Geometry: see drawing. Coordinates: mm, zero at the bounding-box minimum. A direction names the side the tool comes from. Coordinates: 2 decimals unless noted, no trailing zeros. Loops run counter-clockwise (first coordinate to the right, second up) from the corner with the lowest first, then second, coordinate; pieces in that order, holes last. Notation, with made-up numbers: (-26.75, 14.5) -> (-9.75, 14.5) arc R16 ccw to (-9.75, 31.5) -> close; hole circle Ø10 at (-6, 38). An arc over 180 degrees is marked (long way). Answer as a JSON object with one key per item and string values.
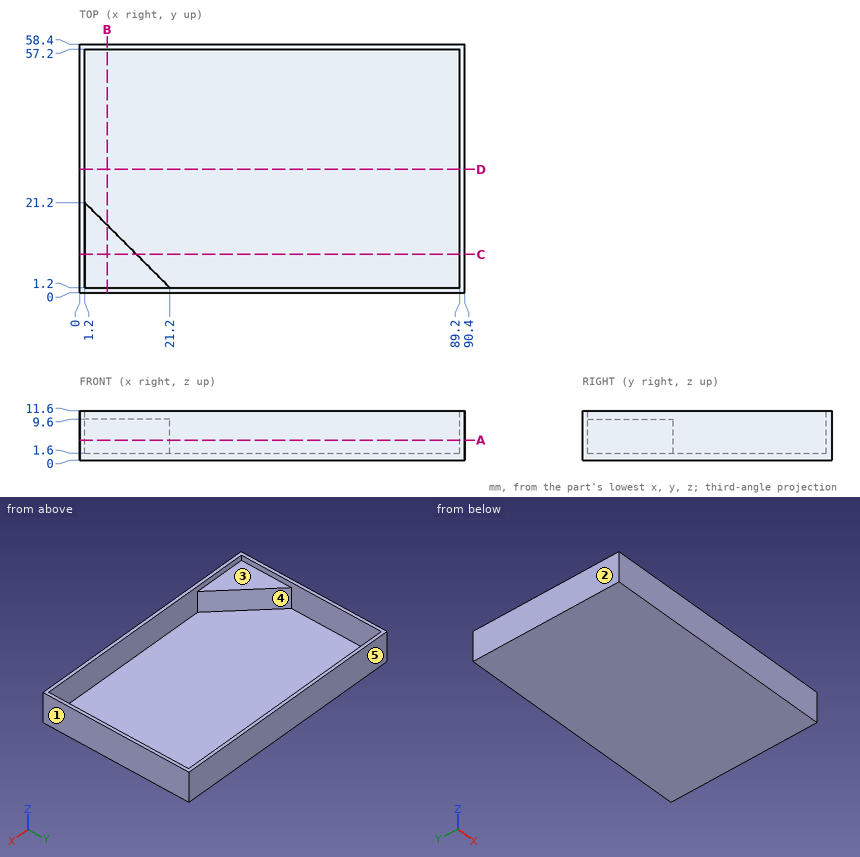
1. Mould query, pull axis X, two halves, no side actions, for the marked faces 1, 2 and 3. Classes: pulls with the +X half, pulls with the -X half, needs draft (parallel to the pull), parting line crosses it, or undercut.
Reply:
{"face 1": "pulls with the +X half", "face 2": "pulls with the -X half", "face 3": "undercut"}
2. Pin query (flat end, axial travel): P1, Ø3, axis at y = 47, z = 4, coming from the -X side; P2, Ø8, axis at x = 43, y = 11, coming from the +Z side; P3, Ø6, axis at x = 8, y = 9, coming from the +Z side. Return the tip coordinate at first contact, or that it passes through.
Reply:
{"P1": "stops at x = 0", "P2": "stops at z = 1.6", "P3": "stops at z = 9.6"}
3. Access query for the marked faces 4 and 5. Directions: +Z, -Z, +X, -X, +Y, -Y. A direction counts if a zero-diameter tool reaches every point of the face in a straight line with its end or side. Return the directions, or none.
Reply:
{"face 4": "+Z", "face 5": "+Z, -Z, +X, -X, +Y"}
4. Line query: line 1 along Y through (x, z) = (43, 9); line 2 along X through (y, z) = (36.5, 5.75); line 3 along Z through (x, y) = (61.5, 39). Output: solid intervals per line, ascending.
Reply:
{"line 1": "y = 0 to 1.2, 57.2 to 58.4", "line 2": "x = 0 to 1.2, 89.2 to 90.4", "line 3": "z = 0 to 1.6"}
5. Section query D-D (y = 29). Return loops of the section in (x, z), plus the area to 3 significant figures.
Reply:
{"outline": "(0, 0) -> (90.4, 0) -> (90.4, 11.6) -> (89.2, 11.6) -> (89.2, 1.6) -> (1.2, 1.6) -> (1.2, 11.6) -> (0, 11.6) -> close", "area": "169 mm2"}
6. Section query C-C (y = 9). Return loops of the section in (x, z), plus the area to 3 significant figures.
Reply:
{"outline": "(0, 0) -> (90.4, 0) -> (90.4, 11.6) -> (89.2, 11.6) -> (89.2, 1.6) -> (13.4, 1.6) -> (13.4, 9.6) -> (1.2, 9.6) -> (1.2, 11.6) -> (0, 11.6) -> close", "area": "266 mm2"}
7. Section query A-A (z = 4.75). Return loops of the section in (x, y).
Reply:
{"outline": "(0, 0) -> (90.4, 0) -> (90.4, 58.4) -> (0, 58.4) -> close; hole (1.2, 21.2) -> (21.2, 1.2) -> (89.2, 1.2) -> (89.2, 57.2) -> (1.2, 57.2) -> close"}
8. Section query B-B (x = 6.5). Return loops of the section in (y, z), plus the area to 3 significant figures.
Reply:
{"outline": "(0, 0) -> (58.4, 0) -> (58.4, 11.6) -> (57.2, 11.6) -> (57.2, 1.6) -> (15.9, 1.6) -> (15.9, 9.6) -> (1.2, 9.6) -> (1.2, 11.6) -> (0, 11.6) -> close", "area": "235 mm2"}
